Here's how the part is built. I have some questions about the finished solid (model axes, mm). Face numbers are marked on the shaded views. A direction names the side the tool comes from. Round coordinates to 2 decimals unless told otherwise and drop trailing zeros. Order: outer loops, then holes, each group sorted by start corner. A loop starts at its lowest first (then second) coordinate and runs counter-clockwise, first axis right, second up. Notation, with made-up numbers: (72, 81) -> (118, 81) arc R17 ccw to (118, 111) -> close; hole circle Ø7 at (63, 18). An arc over 180 degrees is marked (long way). Use a Markdown table: item, result. Add a question column.
(1) I want a section at B-B, the plane y = 12. Please give me the cut outline in (x, z) (3 decimals).
(2) I want a section at D-D, the plane z = 1.5. Please give me the cut outline in (x, y).
(3) On a 3-axis mill with a long thin cutter (end or side, diameter ignored), from which of +Z, -Z, +X, -X, +Y, -Y can I reach the whole of each face in a straight line? I mean the marked faces 1 and 2. Say none if no direction works.
(4) I'm going to push flat-ended pins straight in: P1, Ø3, axis at y = 3.5, z = 4.5, coming from the -X side; P2, Ø10, axis at x = 5, z = 14, coming from the -Y side; P3, Ø6, axis at x = 9, y = 10.5, coming from the +Z side; P4, Ø5, axis at y = 4.5, z = 11.5, coming from the -X side. Where does each tip first touch, or does it pass through?
(5) If I drill on probe 1 along Z at (x, y) = (15.25, 2.5); probe 2 along X at (y, z) = (8, 21.5); probe 3 along X at (y, z) = (1.75, 18.75), over which ranges is the centre line in solid material (lowest first)?
(6) I want a section at C-C, the plane x = 2.75. Please give me the cut outline in (y, z).
from build123d import *

# Parameters (mm, degrees)
SKETCH1_W           = 6.35
SKETCH1_H           = 12.7
BOSS_EXTRUDE1_DEPTH = 2
BOSS_EXTRUDE2_DEPTH = 12.7
SKETCH3_R           = 3.5
CUT_EXTRUDE1_DEPTH  = 13.990381057


with BuildPart() as part:
    # Sketch1 → Boss-Extrude1 (new body)
    with BuildSketch(Plane.XY):
        with Locations((3.175, 6.35)):
            Rectangle(SKETCH1_W, SKETCH1_H)
    extrude(amount=BOSS_EXTRUDE1_DEPTH)

    # Sketch2 → Boss-Extrude2 (add)
    with BuildSketch(Plane.XZ):
        Polygon((6.35, 0), (18.85, 21.650635095), (16.975, 22.733166849), (3.85, 0), align=None)
    extrude(amount=-BOSS_EXTRUDE2_DEPTH)

    # Sketch3 → Cut-Extrude1 (cut, through all)
    with BuildSketch(Plane(origin=(2.8875, 0, -1.667098902), x_dir=(0.5, 0, 0.866025404), z_dir=(-0.866025404, 0, 0.5))):
        with Locations((21.734401077, 6.35)):
            Circle(SKETCH3_R)
    extrude(amount=-CUT_EXTRUDE1_DEPTH, mode=Mode.SUBTRACT)


solid = part.part
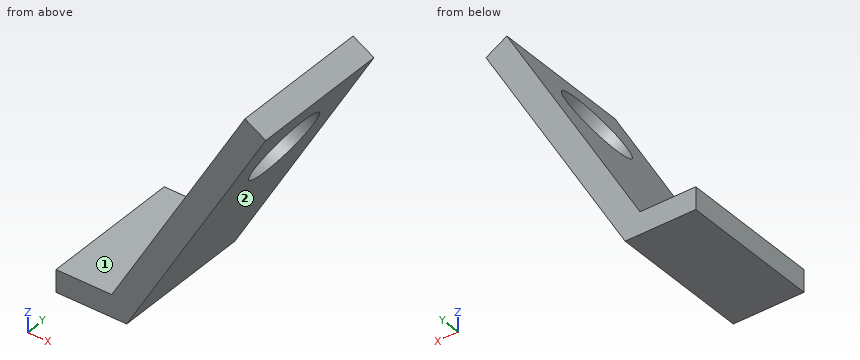
Taken from the geometry:
| question | item | result |
|---|---|---|
| 1 | outline | (0, 0) -> (6.35, 0) -> (18.85, 21.651) -> (16.975, 22.733) -> (5.005, 2) -> (0, 2) -> close |
| 2 | outline | (0, 0) -> (7.22, 0) -> (7.22, 12.7) -> (0, 12.7) -> close |
| 3 | face 1 | +Z, -X, +Y, -Y |
| 3 | face 2 | -Z, +X, +Y, -Y |
| 4 | P1 | stops at x = 5.58 |
| 4 | P2 | passes through |
| 4 | P3 | stops at z = 14.12 |
| 4 | P4 | stops at x = 9.05 |
| 5 | probe 1 | z = 15.42 to 19.75 |
| 5 | probe 2 | x = 16.26 to 18.76 |
| 5 | probe 3 | x = 14.68 to 17.18 |
| 6 | outline | (0, 0) -> (12.7, 0) -> (12.7, 2) -> (0, 2) -> close |
